Can you work these out from the model? Positions are in its coordinate system, mm. A direction names the side the tool comes from. Coordinates: 2 decimals unless noted, no trailing zeros. Write each loop counter-clockwise with the first axis right and the second up, starting at its lowest first coordinate (ties: lowest second). Pieces come first, ordered by that corner, then holes. Notation, with made-up numbers: (-37, -33) -> (20, -33) arc R16 cw to (20, -14) -> close; hole circle Ø3 at (-16.5, 31). An arc over 180 degrees is marked (long way). Use one line per item in the form item = value.
```python
from build123d import *

# Parameters (mm, degrees)
SKETCH_1_R      = 4.5
EXTRUDE_1_DEPTH = 20
EXTRUDE_2_DEPTH = 10
CHAMFER_2_SIZE  = 1
FILLET_1_R      = 2


with BuildPart() as part:
    # 草圖1 → 填料-伸長1 (new body)
    with BuildSketch(Plane(origin=(0, 0, 0), x_dir=(1, 0, 0), z_dir=(0, 1, 0))):
        Circle(SKETCH_1_R)
    extrude(amount=EXTRUDE_1_DEPTH)

    # 草圖2 → 填料-伸長2 (add)
    with BuildSketch(Plane(origin=(0, 20, 0), x_dir=(1, 0, 0), z_dir=(0, 1, 0))):
        Polygon((6, 3.464101615), (0, 6.92820323), (-6, 3.464101615), (-6, -3.464101615), (0, -6.92820323), (6, -3.464101615), align=None)
    extrude(amount=EXTRUDE_2_DEPTH)

    # 導角2
    chamfer_2_edges = [part.edges().sort_by_distance(p)[0] for p in [
        (-4.5, 0, 0),
        (-4.5, 20, 0),
    ]]
    chamfer(chamfer_2_edges, length=CHAMFER_2_SIZE)

    # 圓角1
    fillet_1_edges = [part.edges().sort_by_distance(p)[0] for p in [
        (6, 30, 0),
        (3, 30, -5.196152423),
        (-3, 30, -5.196152423),
        (-6, 30, 0),
        (-3, 30, 5.196152423),
        (3, 30, 5.196152423),
    ]]
    fillet(fillet_1_edges, radius=FILLET_1_R)


solid = part.part
```
Q1. Suppose I cut it at C-C (y = 4.25). Write out the boundary of the cut face in (x, z), then the cut area to 3 significant figures.
Return value:
outline = circle Ø9 at (0, 0)
area = 63.6 mm2
Q2. Suppose I cut it at A-A (z = 0). Write out the boundary of the cut face in (x, y).
Return value:
outline = (-6, 20) -> (-5.5, 20) -> (-4.5, 19) -> (-4.5, 1) -> (-3.5, 0) -> (3.5, 0) -> (4.5, 1) -> (4.5, 19) -> (5.5, 20) -> (6, 20) -> (6, 28) arc R2 ccw to (4, 30) -> (-4, 30) arc R2 ccw to (-6, 28) -> close
Q3. Suppose I cut it at B-B (y = 25). Write out the boundary of the cut face in (x, z), then the cut area to 3 significant figures.
Return value:
outline = (-6, -3.46) -> (0, -6.93) -> (6, -3.46) -> (6, 3.46) -> (0, 6.93) -> (-6, 3.46) -> close
area = 125 mm2
Q4. Will these pins go through, and if not, where does the flat tip stop? pin 1 (6 mm diameter, centred on x = -4, y = 10, fed in from -Z); pin 2 (3 mm diameter, centred on x = 2.5, y = 12, fed in from +Z); pin 3 (3 mm diameter, centred on x = 3, z = -5, fed in from +Y); pin 4 (3 mm diameter, centred on x = 2, z = -3.5, fed in from -Y).
Return value:
pin_1 = -4.39
pin_2 = 4.39
pin_3 = 29.97
pin_4 = 0
Q5. For faces 1 (the cylindrical face through (2.757, 29.399, 4.678)), 2 (the cylindrical face through (-0.59, 9.87, -4.46)), which set-ups out of +Z, -Z, +X, -X, +Y, -Y let a thin tool reach every point of the face, with its end or its side?
Return value:
face_1 = +Z, +X, +Y
face_2 = -Y
Q6. If I drill on line 1 (Z direction, x = 0.25, y = 5.5); line 2 (X direction, y = 23, z = 4.25); line 3 (Z direction, x = -0.25, y = 26), over which ranges is the centre line in solid material (lowest first)? Write a range as from..to.
Return value:
line_1 = -4.49..4.49
line_2 = -4.64..4.64
line_3 = -6.78..6.78
